Read the model definition and answer for the solid it produces. Units are mm, in the model's axes. A direction names the side the tool comes from. Coordinates: 2 decimals unless noted, no trailing zeros. Loops run counter-clockwise (first coordinate to the right, second up) from the corner with the lowest first, then second, coordinate; pieces in that order, holes last. Notation, with made-up numbers: (88.25, -13) -> (109.25, -13) arc R23 cw to (109.25, 9) -> close; hole circle Ø9 at (85.25, 65.5). An arc over 180 degrees is marked (long way). Answer as a JSON object with one key per item and string values. Group by question number.
Q1. Straight lines are drawn through the part: line 1 along Y through (x, z) = (-37, 2); line 2 along X through (y, z) = (-18.5, 20.5); line 3 along Z through (x, y) = (-34, -8). For each, find the intervals that lie inside material, in ascending order. Write a range as [from, to].
Q2. Each of these flat-tipped pins is pushed along its axis until it touches: P1, Ø12, axis at x = -11.5, z = 26, coming from the +Y side; P2, Ø12, axis at x = -36.5, y = -10, coming from the +Z side; P3, Ø5, axis at y = -4.5, z = 31, coming from the -X side. Where does it stop, or does it pass through?
Q3. For faces 1 (the flat face through (-3, 6, 23)), 2 (the flat face through (-1, 0, 35)), determine the directions among +Z, -Z, +X, -X, +Y, -Y from which every point of the face is accessible in a straight line to the end or side of a thin tool.
Q4. The part is cut by section D-D on z = 18. Write down the section's boundary in (x, y), and give its area (3 significant figures).
Q5. The part is cut by section B-B on x = -37.5. Write down the section's boundary in (y, z).
Q6. The part is cut by section A-A on y = 0. Write down the section's boundary in (x, z), and give its area (3 significant figures).
Q7. Determine the mould class of faces 3 (the cylindrical face through (-13.95, -14.3, 1.52)), 4 (the cylindrical face through (-1.128, 0.35, 1.069)), 5 (the flat face through (-17, 25, 2)) for opening direction Y: released by +Y, released by -Y, zero draft, split by the parting line, or undercut.
Q8. The part is cut by section C-C on y = -17. Write down the section's boundary in (x, z), and give its area (3 significant figures).
from build123d import *

# Parameters (mm, degrees)
SM_BASE_FLANGE_1_DEPTH = 25
FILLET_1_R             = 20
SKETCH_8_R             = 8
CUT_EXTRUDE_1_DEPTH    = 63.24949799
SKETCH_9_R             = 4
CUT_EXTRUDE_2_DEPTH    = 61.613529843


# Sheet-metal steps are written as plain solids
with BuildPart() as part:
    # Sketch 1 → Базовая кромка1 (new body)
    with BuildSketch(Plane(origin=(0, 0, 0), x_dir=(1, 0, 0), z_dir=(0, 1, 0))):
        with BuildLine():
            Line((-45, 0), (-3.75, 0))
            ThreePointArc((-3.75, 0), (-1.098349571, -1.098349571), (0, -3.75))
            Line((0, -3.75), (0, -35))
            Line((0, -35), (-3, -35))
            Line((-3, -35), (-3, -3.75))
            ThreePointArc((-3, -3.75), (-3.219669914, -3.219669914), (-3.75, -3))
            Line((-3.75, -3), (-45, -3))
            Line((-45, -3), (-45, 0))
        make_face()
    extrude(amount=SM_BASE_FLANGE_1_DEPTH)

    # Скругление1
    fillet_1_edges = [part.edges().sort_by_distance(p)[0] for p in [
        (-1.5, 25, 35),
    ]]
    fillet(fillet_1_edges, radius=FILLET_1_R)

    # Зеркальное отражение1: part across plane


with BuildPart() as part_1:
    add(part.part)
    add(part.part.mirror(Plane(origin=(-3.75, 0, 3.75), x_dir=(0, 0, 1), z_dir=(0, 1, 0))))

    # Эскиз8 → Вырез-Вытянуть1 (cut, through all)
    with BuildSketch(Plane(origin=(0, 0, 0), x_dir=(0, 0, -1), z_dir=(1, 0, 0))):
        with Locations((-17, 0)):
            Circle(SKETCH_8_R)
    extrude(amount=-CUT_EXTRUDE_1_DEPTH, mode=Mode.SUBTRACT)

    # Эскиз9 → Вырез-Вытянуть2 (cut, through all)
    with BuildSketch(Plane.XY.offset(3)):
        with Locations((-37, 17)):
            Circle(SKETCH_9_R)
        with Locations((-11, 17)):
            Circle(SKETCH_9_R)
        with Locations((-11, -17)):
            Circle(SKETCH_9_R)
        with Locations((-37, -17)):
            Circle(SKETCH_9_R)
    extrude(amount=-CUT_EXTRUDE_2_DEPTH, mode=Mode.SUBTRACT)


solid = part_1.part
Final values:
{
 "1": {"line 1": "y = [-25, -21], [-13, 13], [21, 25]", "line 2": "x = [-3, 0]", "line 3": "z = [0, 3]"},
 "2": {"P1": "passes through", "P2": "stops at z = 3", "P3": "stops at x = -3"},
 "3": {"face 1": "+Z, -X, +Y, -Y", "face 2": "+Z, +X, -X, +Y, -Y"},
 "4": {"outline": "(-3, -24.77) -> (0, -24.77) -> (0, -7.94) -> (-3, -7.94) -> close; (-3, 7.94) -> (0, 7.94) -> (0, 24.77) -> (-3, 24.77) -> close", "area": "101 mm2"},
 "5": {"outline": "(-25, 0) -> (-20.97, 0) -> (-20.97, 3) -> (-25, 3) -> close; (-13.03, 0) -> (13.03, 0) -> (13.03, 3) -> (-13.03, 3) -> close; (20.97, 0) -> (25, 0) -> (25, 3) -> (20.97, 3) -> close"},
 "6": {"outline": "(-45, 0) -> (-3.75, 0) arc R3.75 ccw to (0, 3.75) -> (0, 9) -> (-3, 9) -> (-3, 3.75) arc R0.75 cw to (-3.75, 3) -> (-45, 3) -> close; (-3, 25) -> (0, 25) -> (0, 35) -> (-3, 35) -> close", "area": "180 mm2"},
 "7": {"face 3": "undercut", "face 4": "zero draft", "face 5": "released by +Y"},
 "8": {"outline": "(-45, 0) -> (-41, 0) -> (-41, 3) -> (-45, 3) -> close; (-33, 0) -> (-15, 0) -> (-15, 3) -> (-33, 3) -> close; (-7, 0) -> (-3.75, 0) arc R3.75 ccw to (0, 3.75) -> (0, 31) -> (-3, 31) -> (-3, 3.75) arc R0.75 cw to (-3.75, 3) -> (-7, 3) -> close", "area": "168 mm2"}
}
